Answer from the drawing. Dimensions are ordinates in mm from the lowest x, y and z of the part. A direction names the side the tool comes from. Give positions to 0.01 mm unless a question says otherwise; leave off trailing zeros. Write each loop counter-clockwise with the first axis right and the second up, starting at its lowest first coordinate (ties: lowest second). Pieces come first, ordered by that corner, then holes.
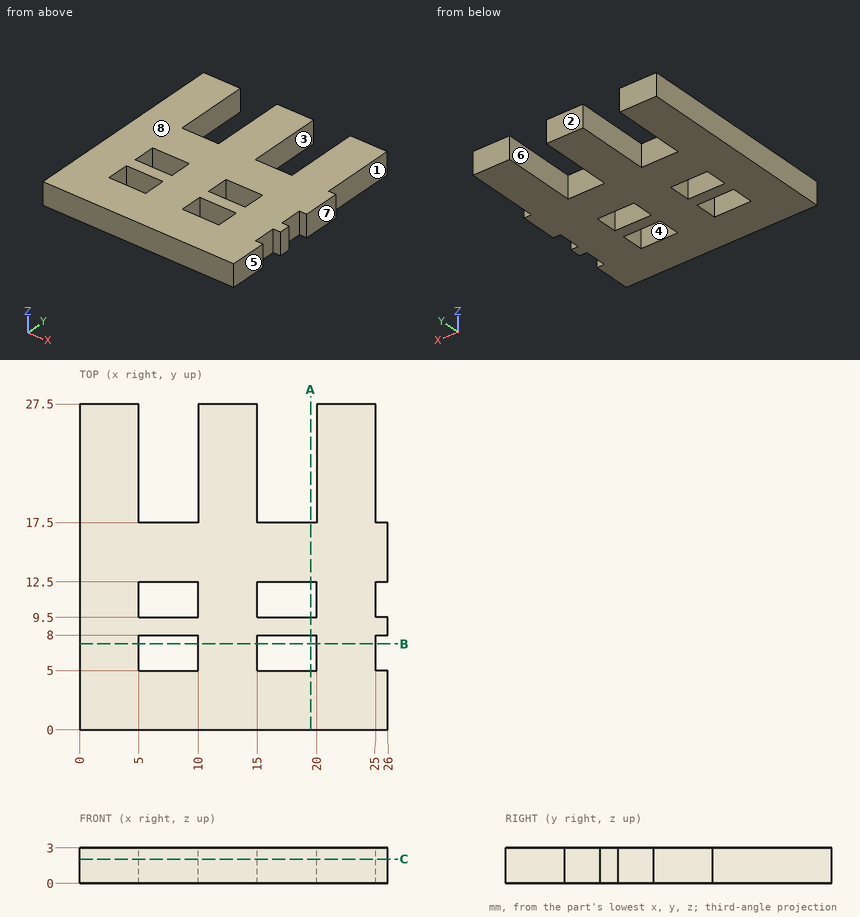
Item 1: A cutting plane is placed at B-B, the plane y = 7.25. Give the vertices of the cut face in (x, z), plus the area to 3 significant figures.
Conclusion:
outline: (0, 0) - (5, 0) - (5, 3) - (0, 3) - close; (10, 0) - (15, 0) - (15, 3) - (10, 3) - close; (20, 0) - (25, 0) - (25, 3) - (20, 3) - close
area: 45.0 mm2
Item 2: Which of the six approach directions +Z, -Z, +X, -X, +Y, -Y give full straight-line access (tool end or side, diameter ignored) to the marked faces 1, 2, 3, 4 and 5?
Conclusion:
face 1: +Z, -Z, +X, +Y
face 2: +Z, -Z, +X, -X, +Y
face 3: +Z, -Z, +Y
face 4: +Z, -Z
face 5: +Z, -Z, +X, +Y, -Y
Item 3: Consider probe 1 along Y at (x, z) = (18, 2.4); probe 2 along X at (y, z) = (6.25, 1.75). Determine where each line is inside the solid, lowest interval first.
Conclusion:
probe 1: y = 0 to 5, 8 to 9.5, 12.5 to 17.5
probe 2: x = 0 to 5, 10 to 15, 20 to 25
Item 4: Determine the mould class of the marked faces 6, 7 and 8 for opening direction X: pulls with the +X half, pulls with the -X half, needs draft (parallel to the pull), parting line crosses it, or undercut.
Conclusion:
face 6: undercut
face 7: pulls with the +X half
face 8: needs draft
Item 5: A cutting plane is placed at A-A, the plane x = 19.5. Give the vertices of the cut face in (y, z), plus the area to 3 significant figures.
Conclusion:
outline: (0, 0) - (5, 0) - (5, 3) - (0, 3) - close; (8, 0) - (9.5, 0) - (9.5, 3) - (8, 3) - close; (12.5, 0) - (17.5, 0) - (17.5, 3) - (12.5, 3) - close
area: 34.5 mm2
Item 6: A cutting plane is placed at C-C, the plane z = 2.05. Count the separate pieces of the cut face and the enclosed holes in it, plus the area to 3 significant figures.
Conclusion:
separate pieces: 1
enclosed holes: 4
area: 539 mm2
Item 7: Each of these flat-tipped pins is pushed along its axis until it touches: P1, Ø2, axis at x = 8, y = 19, coming from the +Z side; P2, Ø0.9, axis at y = 7, z = 1.5, coming from the +X side; P3, Ø1.5, axis at x = 6.5, z = 1, coming from the +Y side. Where does it stop, or does it pass through?
Conclusion:
P1: passes through
P2: stops at x = 25
P3: stops at y = 17.5
